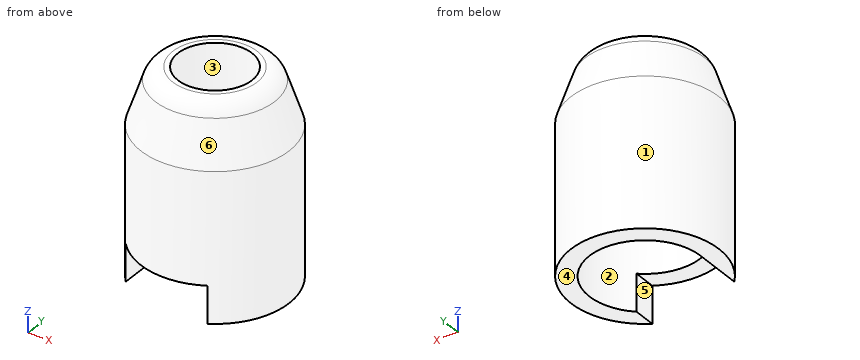
from build123d import *

# Parameters (mm, degrees)
SKETCH1_R           = 4
SKETCH1_R_2         = 3
BOSS_EXTRUDE1_DEPTH = 8
SKETCH2_R           = 4
SKETCH3_R           = 3
SKETCH4_R           = 2
CUT_EXTRUDE1_DEPTH  = 13.369316942
FILLET1_R           = 1
SKETCH5_W           = 5
SKETCH5_H           = 2
CUT_EXTRUDE2_DEPTH  = 6


with BuildPart() as part:
    # Sketch1 → Boss-Extrude1 (new body)
    with BuildSketch(Plane.XY):
        Circle(SKETCH1_R)
        Circle(SKETCH1_R_2, mode=Mode.SUBTRACT)
    extrude(amount=BOSS_EXTRUDE1_DEPTH)

    # Sketch2 → Loft1 section 0
    with BuildSketch(Plane.XY.offset(8)):
        Circle(SKETCH2_R)
    # Sketch3 → Loft1 section 1
    with BuildSketch(Plane.XY.offset(11)):
        Circle(SKETCH3_R)
    loft()

    # Sketch4 → Cut-Extrude1 (cut, through all)
    with BuildSketch(Plane.XY.offset(11)):
        Circle(SKETCH4_R)
    extrude(amount=-CUT_EXTRUDE1_DEPTH, mode=Mode.SUBTRACT)

    # Fillet1
    fillet1_edges = [part.edges().sort_by_distance(p)[0] for p in [
        (-3, 0, 11),
    ]]
    fillet(fillet1_edges, radius=FILLET1_R)

    # Sketch5 → Cut-Extrude2 (cut)
    with BuildSketch(Plane(origin=(0, 0, 0), x_dir=(1, 0, 0), z_dir=(0, 1, 0))):
        with Locations((-0.5, -1)):
            Rectangle(SKETCH5_W, SKETCH5_H)
    extrude(amount=-CUT_EXTRUDE2_DEPTH, mode=Mode.SUBTRACT)


solid = part.part
CAD build for the part. Positions are in the model's coordinates, mm. Face numbers are marked on the shaded views. A direction names the side the tool comes from. Round coordinates to 2 decimals unless told otherwise and drop trailing zeros. Write each loop counter-clockwise with the first axis right and the second up, starting at its lowest first coordinate (ties: lowest second). Pieces come first, ordered by that corner, then holes. Notation, with made-up numbers: M 25,14 L 57,14 A27 ccw 57,49 Z; hole C 70,50 d4. An arc over 180 degrees is marked long. Put each result on its own line as item: value. Start each with the question number.
1) Saw through at A-A, the plane x = 0. Write the cut outline in (y, z), and give its area (3 significant figures).
2) Pull direction X, two halves, no side cores. Call the marked faces 3, 4, 5 and 6: pulls with the +X half, pulls with the -X half, needs draft (parallel to the pull), parting line crosses it, or undercut.
3) Drill centre lines: probe 1 along X at (y, z) = (0, 6.25); probe 2 along Z at (x, y) = (0.25, 2.25). Where is each one in solid material? Low to high. Write a range as [from, to].
4) 3-axis set-ups, long thin cutter, end or side, ignore diameter. For the marked faces 1 and 2: which of +Z, -Z, +X, -X, +Y, -Y reach the whole face in a straight line?
5) Saw through at B-B, the plane z = 1.5. Write the cut outline in (x, y).
6) Pin check, flat tips, straight feed: pin 1 Ø1.5 at (y, z) = (1.5, 6) entering from -X; pin 2 Ø0.6 at (y, z) = (-2.5, 1) entering from -X; pin 3 Ø1.5 at (y, z) = (-1.5, 9) entering from -X; pin 4 Ø2 at (y, z) = (-1, 1) entering from +X. Stop position of each tip, or through.
Resolved:
1. outline: M -4,2 L -3,2 L -3,8 L -2,8 L -2,11 L -2.28,11 A1 ccw -3.23,10.32 L -4,8 Z; M 2,8 L 3,8 L 3,0 L 4,0 L 4,8 L 3.23,10.32 A1 ccw 2.28,11 L 2,11 Z
1. area: 22.8 mm²
2. face 3: undercut
2. face 4: needs draft
2. face 5: undercut
2. face 6: parting line crosses it
3. probe 1: [-4, -3], [3, 4]
3. probe 2: [8, 11]
4. face 1: +Z, -Z
4. face 2: -Z
5. outline: M -3,-2.65 L -3,0 A3 cw long 2,-2.24 L 2,-3.46 A4 ccw long Z
6. pin 1: x = -3.93
6. pin 2: x = -3.34
6. pin 3: x = -3.72
6. pin 4: x = 4
